The figure shows three views and two pictorial views of one solid part (mm, origin at its lowest corner). Answer the questions. A direction names the side the tool comes from. Coordinates: 2 decimals unless noted, no trailing zeros. Loops run counter-clockwise (first coordinate to the right, second up) from the corner with the lowest first, then second, coordinate; pieces in that order, holes last. Notation, with made-up numbers: (76.5, 51) -> (101.5, 51) arc R15 cw to (101.5, 69) -> close; hole circle Ø11 at (-18, -4). An arc over 180 degrees is marked (long way). Answer in a Markdown table with one row per item.
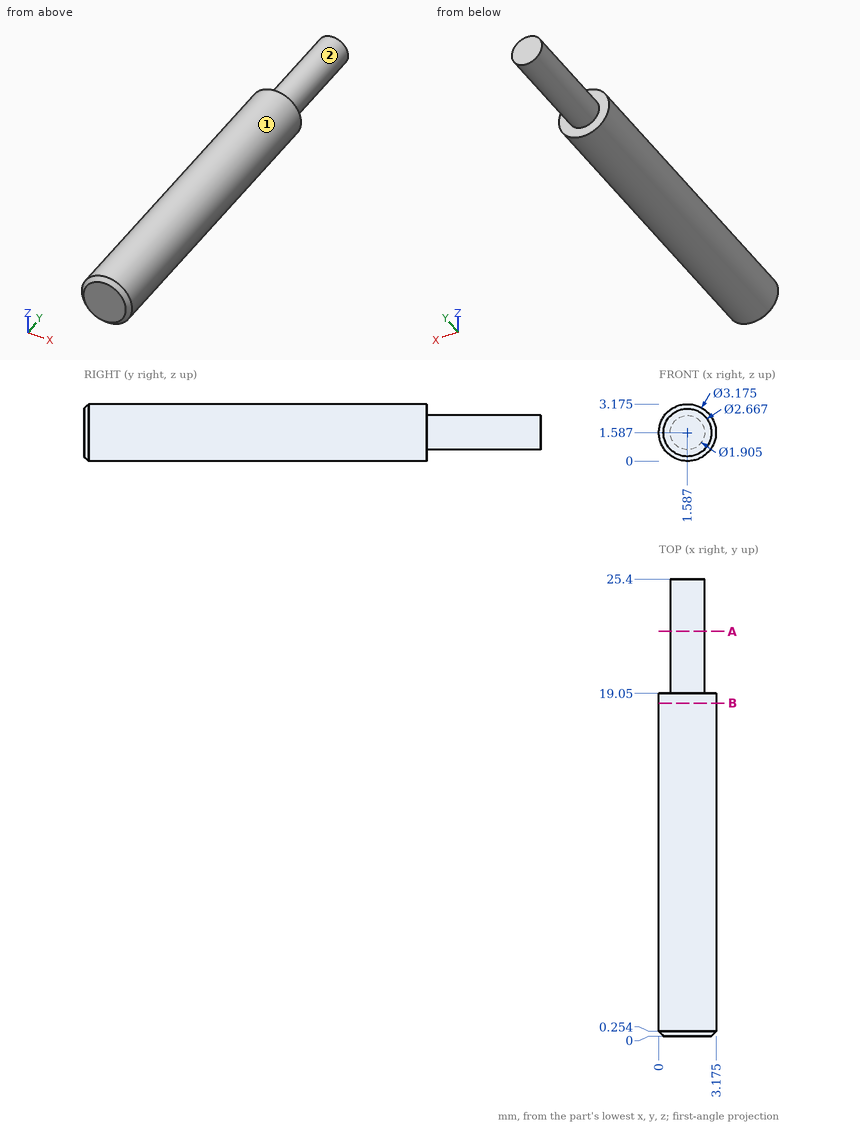
Item 1: A cutting plane is placed at A-A, the plane y = 22.5. Determine the outline of the cut face in (x, z) (1 decimal).
Findings below:
| item | result |
|---|---|
| outline | circle Ø1.9 at (1.6, 1.6) |
Item 2: Flat-ended cylindrical pins translate along their axes: pin 1 Ø1.5 at (y, z) = (14.5, 0.5) entering from -X; pin 2 Ø1.5 at (x, y) = (2.5, 5) entering from +Z. Find the tip coordinate at first contact, or state that the pin passes through.
Findings below:
| item | result |
|---|---|
| pin 1 | stops at x = 0.04 |
| pin 2 | stops at z = 3.17 |
Item 3: A cutting plane is placed at B-B, the plane y = 18.5. Determine the outline of the cut face in (x, z) (1 decimal).
Findings below:
| item | result |
|---|---|
| outline | circle Ø3.2 at (1.6, 1.6) |
Item 4: A tool of negligible diameter and unlimited length cuts with its end or side. For the marked faces 1 and 2, from which of +Z, -Z, +X, -X, +Y, -Y can it reach the whole face along a straight path? Write none if from no direction.
Findings below:
| item | result |
|---|---|
| face 1 | +Y, -Y |
| face 2 | +Y |
Item 5: Find the intervals of material crossed by probe 1 along Y at (x, z) = (0.6, 2.2); probe 2 along Z at (x, y) = (2.45, 1.5) (1 decimal); probe 3 along Z at (x, y) = (1.7, 3) (1 decimal), in increasing order.
Findings below:
| item | result |
|---|---|
| probe 1 | y = 0 to 19.05 |
| probe 2 | z = 0.3 to 2.9 |
| probe 3 | z = 0 to 3.2 |
